```python
from build123d import *

# Parameters (mm, degrees)
BOSS_EXTRUDE1_DEPTH      = 140.208
BOSS_EXTRUDE1_DEPTH_BACK = 164.338


with BuildPart() as part:
    # First Part → Boss-Extrude1 (new, two sides: drawn at the far end of the back side and taken through both)
    with BuildSketch(Plane.XY.offset(-BOSS_EXTRUDE1_DEPTH_BACK)):
        with BuildLine():
            Line((0, 0), (0, 76.2))
            Line((0, 76.2), (101.6, 76.2))
            Line((101.6, 76.2), (101.6, -76.2))
            ThreePointArc((101.6, -76.2), (76.2, -101.6), (50.8, -76.2))
            Line((50.8, -76.2), (-76.2, -76.2))
            Line((-76.2, -76.2), (-76.2, 0))
            ThreePointArc((-76.2, 0), (-50.8, 25.4), (-25.4, 0))
            Line((-25.4, 0), (0, 0))
        make_face()
    extrude(amount=BOSS_EXTRUDE1_DEPTH + BOSS_EXTRUDE1_DEPTH_BACK)


solid = part.part
```
Input: part model. Units: mm. Frame: model coordinates. A direction names the side the tool comes from. Coordinates: 2 decimals unless noted, no trailing zeros. Loops run counter-clockwise (first coordinate to the right, second up) from the corner with the lowest first, then second, coordinate; pieces in that order, holes last. Notation, with made-up numbers: (28.5, 81.5) - (42.5, 81.5) arc R26 ccw to (42.5, 106.5) - close; hole circle Ø6 at (6.5, -39). An arc over 180 degrees is marked (long way). Answer in a Markdown table with one row per item.
(1) Set-up query: faces 1 (the face through (-12, -76.2, -14)), 2 (the face through (-13, 0, -14)), 3 (the face through (34, -11, -164.338)). Return all of +Z, -Z, +X, -X, +Y, -Y with unobstructed straight access to the full face (end or side cutting, diameter ignored); none if empty.
Model answer:
| item | result |
|---|---|
| face 1 | +Z, -Z, -X, -Y |
| face 2 | +Z, -Z, +Y |
| face 3 | -Z, +X, -X, +Y, -Y |
(2) Cut plane A-A on y = 12.5. Output: boundary loops of the cut face in (x, z).
Model answer:
| item | result |
|---|---|
| outline | (-72.91, -164.34) - (-28.69, -164.34) - (-28.69, 140.21) - (-72.91, 140.21) - close; (0, -164.34) - (101.6, -164.34) - (101.6, 140.21) - (0, 140.21) - close |
(3) Material intervals for L1, parallel to X at y = 56, z = 13; L2, parallel to Y at x = 38, z = -24; L3, parallel to X at y = 18.5, z = -21, sorted ascending. Write a range as from..to.
Model answer:
| item | result |
|---|---|
| L1 | x = 0..101.6 |
| L2 | y = -76.2..76.2 |
| L3 | x = -68.2..-33.4, 0..101.6 |
(4) Pin query (flat end, axial travel): P1, Ø4, axis at y = 27.5, z = -32.5, coming from the -X side; P2, Ø1, axis at x = -45.5, z = -118.5, coming from the -Y side; P3, Ø2, axis at x = -56, z = 100.5, coming from the +Y side. Return the tip coordinate at first contact, or that it passes through.
Model answer:
| item | result |
|---|---|
| P1 | stops at x = 0 |
| P2 | stops at y = -76.2 |
| P3 | stops at y = 25.05 |
(5) Mould query, pull axis X, two halves, no side actions, for faces 4 (the face through (-51.359, 25.394, -14.197)), 5 (the face through (50, 76.2, -14)), 6 (the face through (76.759, -101.594, -14.197)). Classes: pulls with the +X half, pulls with the -X half, needs draft (parallel to the pull), parting line crosses it, or undercut.
Model answer:
| item | result |
|---|---|
| face 4 | undercut |
| face 5 | needs draft |
| face 6 | parting line crosses it |
(6) Cut plane B-B on z = -72. Output: boundary loops of the cut face in (x, y), plus the area to 3 significant figures.
Model answer:
| item | result |
|---|---|
| outline | (-76.2, -76.2) - (50.8, -76.2) arc R25.4 ccw to (101.6, -76.2) - (101.6, 76.2) - (0, 76.2) - (0, 0) - (-25.4, 0) arc R25.4 ccw to (-76.2, 0) - close |
| area | 23,300 mm² |
(7) Cut plane C-C on y = 62. Output: boundary loops of the cut face in (x, z), plus the area to 3 significant figures.
Model answer:
| item | result |
|---|---|
| outline | (0, -164.34) - (101.6, -164.34) - (101.6, 140.21) - (0, 140.21) - close |
| area | 30,900 mm² |
(8) Cut plane D-D on x = -7. Output: boundary loops of the cut face in (y, z), plus the area to 3 significant figures.
Model answer:
| item | result |
|---|---|
| outline | (-76.2, -164.34) - (0, -164.34) - (0, 140.21) - (-76.2, 140.21) - close |
| area | 23,200 mm² |
